```python
from build123d import *

# Parameters (mm, degrees)
F0_W      = 203.2
F0_H      = 101.6
F1_DEPTH  = 76.2
F2_W      = 50.8
F2_H      = 50.8
F3_DEPTH  = 76.2
F4_W      = 50.8
F4_H      = 25.4
F5_DEPTH  = 50.8
F6_W      = 152.4
F6_H      = 25.4
F7_DEPTH  = 50.8
F8_W      = 50.8
F8_H      = 50.8
F9_DEPTH  = 76.2
F10_W     = 203.2
F10_H     = 50.8
F11_DEPTH = 25.4
F12_R     = 25.4
F13_R     = 25.4
F14_R     = 12.147807
F15_DEPTH = 76.2
F16_R     = 12.7
F17_DEPTH = 50.801


with BuildPart() as f1:
    # F0 (on Top) → F1 (new body)
    with BuildSketch(Plane.XY):
        with Locations((-52.603766, -35.422396)):
            Rectangle(F0_W, F0_H)
    extrude(amount=F1_DEPTH)

    # F2 (on face) → F3 (cut)
    with BuildSketch(Plane.XZ.offset(86.222396)):
        with Locations((23.596234, 25.4)):
            Rectangle(F2_W, F2_H)
    extrude(amount=-F3_DEPTH, mode=Mode.SUBTRACT)

    # F4 (on face) → F5 (cut)
    with BuildSketch(Plane.XZ.offset(86.222396)):
        with Locations((23.596234, 63.5)):
            Rectangle(F4_W, F4_H)
    extrude(amount=-F5_DEPTH, mode=Mode.SUBTRACT)

    # F6 (on face) → F7 (cut)
    with BuildSketch(Plane.XZ.offset(86.222396)):
        with Locations((-78.003766, 63.5)):
            Rectangle(F6_W, F6_H)
    extrude(amount=-F7_DEPTH, mode=Mode.SUBTRACT)

    # F8 (on face) → F9 (cut)
    with BuildSketch(Plane.XZ.offset(86.222396)):
        with Locations((-128.803766, 25.4)):
            Rectangle(F8_W, F8_H)
    extrude(amount=-F9_DEPTH, mode=Mode.SUBTRACT)

    # F10 (on face) → F11 (join)
    with BuildSketch(Plane.XY.offset(76.2)):
        with Locations((-52.603766, -10.022396)):
            Rectangle(F10_W, F10_H)
    extrude(amount=F11_DEPTH)

    # F12
    f12_edges = [f1.edges().sort_by_distance(p)[0] for p in [
        (-154.203766, -10.022396, 101.6),
    ]]
    fillet(f12_edges, radius=F12_R)

    # F13
    f13_edges = [f1.edges().sort_by_distance(p)[0] for p in [
        (48.996234, -10.022396, 101.6),
    ]]
    fillet(f13_edges, radius=F13_R)

    # F14 (on face) → F15 (cut)
    with BuildSketch(Plane.XZ.offset(35.422396)):
        with Locations((-128.803766, 76.2)):
            Circle(F14_R)
    extrude(amount=-F15_DEPTH, mode=Mode.SUBTRACT)

    # F16 (on face) → F17 (cut, through all)
    with BuildSketch(Plane.XZ.offset(35.422396)):
        with Locations((23.596234, 76.2)):
            Circle(F16_R)
    extrude(amount=-F17_DEPTH, mode=Mode.SUBTRACT)


solid = f1.part
```
Build history of the part. All positions in model axes, mm. A direction names the side the tool comes from. Round coordinates to 2 decimals unless told otherwise and drop trailing zeros. Write each loop counter-clockwise with the first axis right and the second up, starting at its lowest first coordinate (ties: lowest second). Pieces come first, ordered by that corner, then holes.
1) Band-saw the part on A-A, the plane y = -24. List the corners of the cut face in (x, z), and give its area (3 significant figures).
2) Band-saw the part on C-C, the plane x = 14. List the corners of the cut face in (y, z).
3) Band-saw the part on D-D, the plane x = -21. List the corners of the cut face in (y, z).
4) 3-axis set-ups, long thin cutter, end or side, ignore diameter. For faces 4 (the flat face through (23, -23, 50.8)), 5 (the flat face through (-54, -35.422, 76)), 6 (the flat face through (-129, -10.022, 26)): which of +Z, -Z, +X, -X, +Y, -Y reach the whole face in a straight line?
5) Drill centre lines: probe 1 along X at (y, z) = (-7, 76); probe 2 along Z at (x, y) = (23.5, -30); probe 3 along Z at (x, y) = (-25.5, -38). Where is each one in solid material? Low to high.
6) Pin check, flat tips, straight feed: pin 1 (7.5 mm diameter, centred on x = -116.5, y = -19.5, fed in from -Z); pin 2 (10 mm diameter, centred on x = -18, z = 69.5, fed in from -Y); pin 3 (1 mm diameter, centred on y = -17, z = 17.5, fed in from +X); pin 4 (20.5 mm diameter, centred on x = 23.6, z = 76.2, fed in from +Y). Stop position of each tip, or through.
7) Band-saw the part on B-B, the plane z = 34. List the corners of the cut face in (x, y).
8) Mould opens along X. For faces 1 (the cylindrical face through (20.843, -10.378, 63.802)), 2 (the flat face through (-54, 15.378, 50)), 3 (the cylindrical face through (41.358, -9.667, 94.357)) say: +X half, -X half, draft (parallel to the pull), parting line (faces both ways), or undercut.
Ans:
1. outline: (-154.2, 50.8) - (-103.4, 50.8) - (-103.4, 0) - (-1.8, 0) - (-1.8, 50.8) - (49, 50.8) - (49, 76.2) arc R25.4 ccw to (23.6, 101.6) - (-128.8, 101.6) arc R25.4 ccw to (-154.2, 76.2) - close; hole circle Ø24.3 at (-128.8, 76.2); hole circle Ø25.4 at (23.6, 76.2)
1. area: 14,200 mm2
2. outline: (-35.42, 50.8) - (-10.02, 50.8) - (-10.02, 0) - (15.38, 0) - (15.38, 67.88) - (-35.42, 67.88) - close; (-35.42, 84.52) - (15.38, 84.52) - (15.38, 101.6) - (-35.42, 101.6) - close
3. outline: (-86.22, 0) - (15.38, 0) - (15.38, 101.6) - (-35.42, 101.6) - (-35.42, 50.8) - (-86.22, 50.8) - close
4. face 4: -Z, +X, -Y
4. face 5: +Z, +X, -X, -Y
4. face 6: -Z, -X, -Y
5. probe 1: x = -154.2 to -140.95, -116.66 to 10.9, 36.29 to 49
5. probe 2: z = 50.8 to 63.5, 88.9 to 101.6
5. probe 3: z = 0 to 50.8
6. pin 1: stops at z = 50.8
6. pin 2: stops at y = -35.42
6. pin 3: stops at x = -1.8
6. pin 4: passes through
7. outline: (-154.2, -10.02) - (-103.4, -10.02) - (-103.4, -86.22) - (-1.8, -86.22) - (-1.8, -10.02) - (49, -10.02) - (49, 15.38) - (-154.2, 15.38) - close
8. face 1: undercut
8. face 2: draft
8. face 3: +X half
